Check sheet for the drawn part. Datum: minimum x, y, z corner. Units: mm. A direction names the side the tool comes from. Coordinates: 2 decimals unless noted, no trailing zeros. Write each loop counter-clockwise with the first axis right and the second up, starting at its lowest first coordinate (ties: lowest second). Pieces come first, ordered by that corner, then holes. Notation, with made-up numbers: (77, -15) -> (89, -15) arc R24 cw to (89, 24) -> close; hole circle Ø8 at (-23, -37). An arc over 180 degrees is marked (long way). Write item = value, one per line. Start each with the question number.
(1) Gauge pin test, flat ends, axial feed: pin 1 Ø4.5 at (x, z) = (29.5, 15.5) entering from -Y; pin 2 Ø3 at (y, z) = (4, 11) entering from -X; pin 3 Ø1.8 at (y, z) = (3, 10) entering from +X. Record the tip position at first contact, or that the pin passes through.
(2) Section check A-A (z = 25.65). Record the cut outline in (x, y).
(3) Section check D-D (y = 2.25). Record the cut outline in (x, z), plus the area to 3 significant figures.
(4) Material ranges on probe 1 along X at (y, z) = (10.7, 4.35); probe 2 along Z at (x, y) = (57.75, 9.1); probe 3 along Y at (x, z) = (33.65, 22.35), recorded low to high. Write a range as [from, to].
(5) Mould release check, pull along X, two halves, no side actions. Record for the marked faces 5, 6 and 7: released by +X, released by -X, zero draft, split by the parting line, or undercut.
(6) Set-up check for the marked faces 1, 2, 3 and 4: record each of +Z, -Z, +X, -X, +Y, -Y from which the full face is reachable in a straight line by a thin tool's end or side.
(7) Section check B-B (y = 11.25). Record the cut outline in (x, z).
(8) Section check C-C (x = 57.75). Record the cut outline in (y, z).
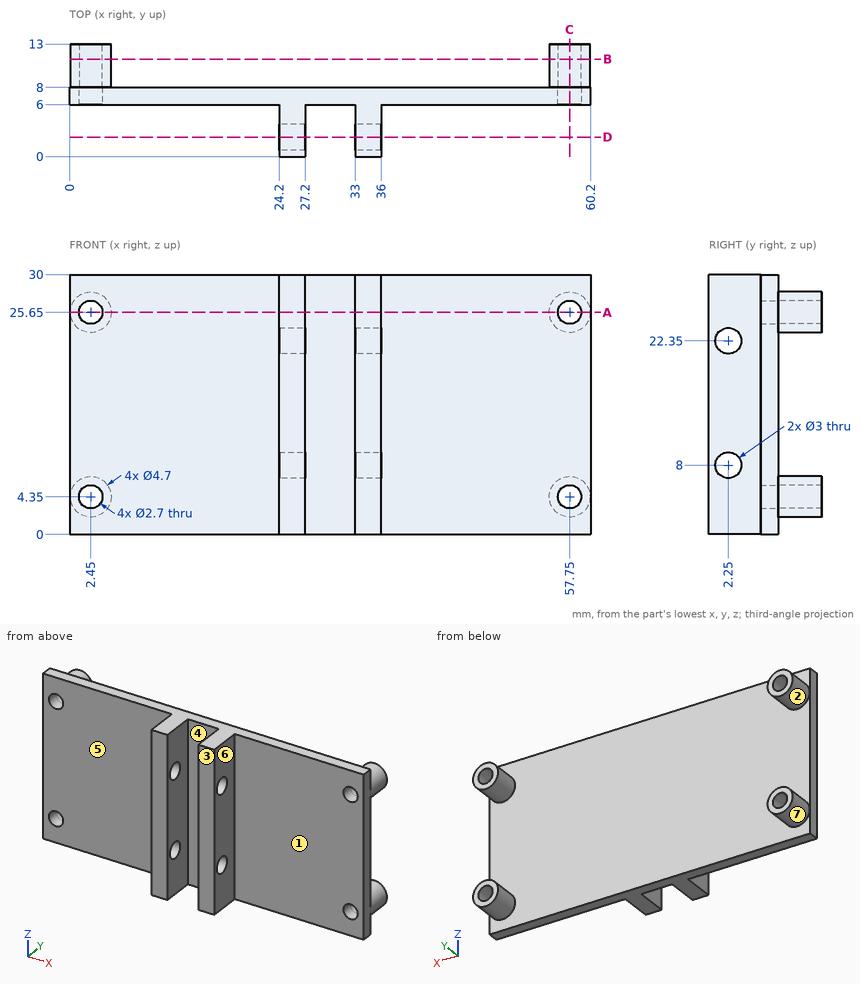
Response:
q1.pin_1 = 6
q1.pin_2 = 24.2
q1.pin_3 = 36
q2.outline = (0, 6) -> (1.1, 6) -> (1.1, 13) -> (0.1, 13) -> (0.1, 8) -> (0, 8) -> close; (3.8, 6) -> (24.2, 6) -> (24.2, 0) -> (27.2, 0) -> (27.2, 6) -> (33, 6) -> (33, 0) -> (36, 0) -> (36, 6) -> (56.4, 6) -> (56.4, 13) -> (55.4, 13) -> (55.4, 8) -> (4.8, 8) -> (4.8, 13) -> (3.8, 13) -> close; (59.1, 6) -> (60.2, 6) -> (60.2, 8) -> (60.1, 8) -> (60.1, 13) -> (59.1, 13) -> close
q3.outline = (24.2, 0) -> (27.2, 0) -> (27.2, 6.5) -> (24.2, 6.5) -> close; (24.2, 9.5) -> (27.2, 9.5) -> (27.2, 20.85) -> (24.2, 20.85) -> close; (24.2, 23.85) -> (27.2, 23.85) -> (27.2, 30) -> (24.2, 30) -> close; (33, 0) -> (36, 0) -> (36, 6.5) -> (33, 6.5) -> close; (33, 9.5) -> (36, 9.5) -> (36, 20.85) -> (33, 20.85) -> close; (33, 23.85) -> (36, 23.85) -> (36, 30) -> (33, 30) -> close
q3.area = 144 mm2
q4.probe_1 = [0.1, 1.1], [3.8, 4.8], [55.4, 56.4], [59.1, 60.1]
q4.probe_2 = [2, 3], [5.7, 6.7], [23.3, 24.3], [27, 28]
q4.probe_3 = [0, 0.75], [3.75, 8]
q5.face_5 = zero draft
q5.face_6 = released by +X
q5.face_7 = undercut
q6.face_1 = +Z, -Z, +X, -Y
q6.face_2 = +Y
q6.face_3 = +Z, -Z, +X, -X, -Y
q6.face_4 = +Z, -Z, -Y
q7.outline = circle Ø4.7 at (2.45, 4.35); circle Ø4.7 at (2.45, 25.65); circle Ø4.7 at (57.75, 4.35); circle Ø4.7 at (57.75, 25.65); hole circle Ø2.7 at (2.45, 4.35); hole circle Ø2.7 at (2.45, 25.65); hole circle Ø2.7 at (57.75, 4.35); hole circle Ø2.7 at (57.75, 25.65)
q8.outline = (6, 0) -> (8, 0) -> (8, 2) -> (13, 2) -> (13, 3) -> (6, 3) -> close; (6, 5.7) -> (13, 5.7) -> (13, 6.7) -> (8, 6.7) -> (8, 23.3) -> (13, 23.3) -> (13, 24.3) -> (6, 24.3) -> close; (6, 27) -> (13, 27) -> (13, 28) -> (8, 28) -> (8, 30) -> (6, 30) -> close
